```python
from build123d import *
from build123d import SkipClean  # not in build123d's __all__

# Parameters (mm, degrees)
F1_DEPTH = 25
F0_R     = 3
F2_DEPTH = 4
F3_SIZE2 = 24.99999
F3_SIZE  = 19.99999
F4_R     = 1


# Not quite as in the source:
# - a fillet or chamfer is up to 0.001 mm smaller than in the source, because OpenCascade refuses the exact size


with BuildPart() as f1:
    # F0 (on Top) → F1 (new body)
    with BuildSketch(Plane.XY):
        with BuildLine():
            ThreePointArc((2, 16.6805275696), (11.8793939239, 11.8793939239), (16.6805275696, 2))
            Line((16.6805275696, 2), (19.6987309236, 2))
            ThreePointArc((19.6987309236, 2), (14.0007142675, 14.0007142675), (2, 19.6987309236))
            Line((2, 19.6987309236), (2, 16.6805275696))
        make_face()
        with BuildLine():
            ThreePointArc((-2, 16.6805275696), (0, 16.8), (2, 16.6805275696))
            Line((2, 16.6805275696), (2, 19.6987309236))
            ThreePointArc((2, 19.6987309236), (0, 19.8), (-2, 19.6987309236))
            Line((-2, 19.6987309236), (-2, 16.6805275696))
        make_face()
        with BuildLine():
            ThreePointArc((-16.6805275696, 2), (-11.8793939239, 11.8793939239), (-2, 16.6805275696))
            Line((-2, 16.6805275696), (-2, 19.6987309236))
            ThreePointArc((-2, 19.6987309236), (-14.0007142675, 14.0007142675), (-19.6987309236, 2))
            Line((-19.6987309236, 2), (-16.6805275696, 2))
        make_face()
        with BuildLine():
            ThreePointArc((-16.6805275696, -2), (-16.8, 0), (-16.6805275696, 2))
            Line((-16.6805275696, 2), (-19.6987309236, 2))
            ThreePointArc((-19.6987309236, 2), (-19.8, 0), (-19.6987309236, -2))
            Line((-19.6987309236, -2), (-16.6805275696, -2))
        make_face()
        with BuildLine():
            Line((-2, -19.6987309236), (-2, -16.6805275696))
            ThreePointArc((-2, -16.6805275696), (-11.8793939239, -11.8793939239), (-16.6805275696, -2))
            Line((-16.6805275696, -2), (-19.6987309236, -2))
            ThreePointArc((-19.6987309236, -2), (-14.0007142675, -14.0007142675), (-2, -19.6987309236))
        make_face()
        with BuildLine():
            Line((2, -19.6987309236), (2, -16.6805275696))
            ThreePointArc((2, -16.6805275696), (0, -16.8), (-2, -16.6805275696))
            Line((-2, -16.6805275696), (-2, -19.6987309236))
            ThreePointArc((-2, -19.6987309236), (0, -19.8), (2, -19.6987309236))
        make_face()
        with BuildLine():
            Line((19.6987309236, -2), (16.6805275696, -2))
            ThreePointArc((16.6805275696, -2), (11.8793939239, -11.8793939239), (2, -16.6805275696))
            Line((2, -16.6805275696), (2, -19.6987309236))
            ThreePointArc((2, -19.6987309236), (14.0007142675, -14.0007142675), (19.6987309236, -2))
        make_face()
        with BuildLine():
            ThreePointArc((16.6805275696, 2), (16.7701052944, 1.0017826188), (16.8, 0))
            ThreePointArc((16.8, 0), (16.7701052944, -1.0017826188), (16.6805275696, -2))
            Line((16.6805275696, -2), (19.6987309236, -2))
            ThreePointArc((19.6987309236, -2), (19.7746665242, -1.0012811076), (19.8, 0))
            ThreePointArc((19.8, 0), (19.7746665242, 1.0012811076), (19.6987309236, 2))
            Line((19.6987309236, 2), (16.6805275696, 2))
        make_face()
        with BuildLine():
            ThreePointArc((-19.6987309236, -2), (-19.8, 0), (-19.6987309236, 2))
            Line((-19.6987309236, 2), (-39.9499687109, 2))
            ThreePointArc((-39.9499687109, 2), (-39.9874902215, 1.0003128423), (-40, 0))
            ThreePointArc((-40, 0), (-39.9874902215, -1.0003128423), (-39.9499687109, -2))
            Line((-39.9499687109, -2), (-19.6987309236, -2))
        make_face()
        with BuildLine():
            Line((2, -39.9499687109), (2, -19.6987309236))
            ThreePointArc((2, -19.6987309236), (0, -19.8), (-2, -19.6987309236))
            Line((-2, -19.6987309236), (-2, -39.9499687109))
            ThreePointArc((-2, -39.9499687109), (-1.0003128423, -39.9874902215), (0, -40))
            ThreePointArc((0, -40), (1.0003128423, -39.9874902215), (2, -39.9499687109))
        make_face()
        with BuildLine():
            Line((39.9499687109, 2), (19.6987309236, 2))
            ThreePointArc((19.6987309236, 2), (19.7746665242, 1.0012811076), (19.8, 0))
            ThreePointArc((19.8, 0), (19.7746665242, -1.0012811076), (19.6987309236, -2))
            Line((19.6987309236, -2), (39.9499687109, -2))
            ThreePointArc((39.9499687109, -2), (39.9874902215, -1.0003128423), (40, 0))
            ThreePointArc((40, 0), (39.9874902215, 1.0003128423), (39.9499687109, 2))
        make_face()
        with BuildLine():
            ThreePointArc((-2, 19.6987309236), (0, 19.8), (2, 19.6987309236))
            Line((2, 19.6987309236), (2, 39.9499687109))
            ThreePointArc((2, 39.9499687109), (1.0003128423, 39.9874902215), (0, 40))
            ThreePointArc((0, 40), (-1.0003128423, 39.9874902215), (-2, 39.9499687109))
            Line((-2, 39.9499687109), (-2, 19.6987309236))
        make_face()
    extrude(amount=F1_DEPTH)

    # F0 (on Top) → F2 (join)
    with BuildSketch(Plane.XY):
        with BuildLine():
            ThreePointArc((-19.6987309236, 2), (-14.0007142675, 14.0007142675), (-2, 19.6987309236))
            Line((-2, 19.6987309236), (-2, 39.9499687109))
            ThreePointArc((-2, 39.9499687109), (-28.2842712475, 28.2842712475), (-39.9499687109, 2))
            Line((-39.9499687109, 2), (-19.6987309236, 2))
        make_face()
        with Locations((-21, 21)):
            Circle(F0_R, mode=Mode.SUBTRACT)
        with BuildLine():
            ThreePointArc((2, 19.6987309236), (14.0007142675, 14.0007142675), (19.6987309236, 2))
            Line((19.6987309236, 2), (39.9499687109, 2))
            ThreePointArc((39.9499687109, 2), (28.2842712475, 28.2842712475), (2, 39.9499687109))
            Line((2, 39.9499687109), (2, 19.6987309236))
        make_face()
        with Locations((21, 21)):
            Circle(F0_R, mode=Mode.SUBTRACT)
        with BuildLine():
            Line((39.9499687109, 2), (19.6987309236, 2))
            ThreePointArc((19.6987309236, 2), (19.7746665242, 1.0012811076), (19.8, 0))
            ThreePointArc((19.8, 0), (19.7746665242, -1.0012811076), (19.6987309236, -2))
            Line((19.6987309236, -2), (39.9499687109, -2))
            ThreePointArc((39.9499687109, -2), (39.9874902215, -1.0003128423), (40, 0))
            ThreePointArc((40, 0), (39.9874902215, 1.0003128423), (39.9499687109, 2))
        make_face()
        with BuildLine():
            ThreePointArc((-2, 19.6987309236), (0, 19.8), (2, 19.6987309236))
            Line((2, 19.6987309236), (2, 39.9499687109))
            ThreePointArc((2, 39.9499687109), (1.0003128423, 39.9874902215), (0, 40))
            ThreePointArc((0, 40), (-1.0003128423, 39.9874902215), (-2, 39.9499687109))
            Line((-2, 39.9499687109), (-2, 19.6987309236))
        make_face()
        with BuildLine():
            Line((39.9499687109, -2), (19.6987309236, -2))
            ThreePointArc((19.6987309236, -2), (14.0007142675, -14.0007142675), (2, -19.6987309236))
            Line((2, -19.6987309236), (2, -39.9499687109))
            ThreePointArc((2, -39.9499687109), (28.2842712475, -28.2842712475), (39.9499687109, -2))
        make_face()
        with Locations((21, -21)):
            Circle(F0_R, mode=Mode.SUBTRACT)
        with BuildLine():
            Line((19.6987309236, -2), (16.6805275696, -2))
            ThreePointArc((16.6805275696, -2), (11.8793939239, -11.8793939239), (2, -16.6805275696))
            Line((2, -16.6805275696), (2, -19.6987309236))
            ThreePointArc((2, -19.6987309236), (14.0007142675, -14.0007142675), (19.6987309236, -2))
        make_face()
        with BuildLine():
            ThreePointArc((16.6805275696, 2), (16.7701052944, 1.0017826188), (16.8, 0))
            ThreePointArc((16.8, 0), (16.7701052944, -1.0017826188), (16.6805275696, -2))
            Line((16.6805275696, -2), (19.6987309236, -2))
            ThreePointArc((19.6987309236, -2), (19.7746665242, -1.0012811076), (19.8, 0))
            ThreePointArc((19.8, 0), (19.7746665242, 1.0012811076), (19.6987309236, 2))
            Line((19.6987309236, 2), (16.6805275696, 2))
        make_face()
        with BuildLine():
            ThreePointArc((2, 16.6805275696), (11.8793939239, 11.8793939239), (16.6805275696, 2))
            Line((16.6805275696, 2), (19.6987309236, 2))
            ThreePointArc((19.6987309236, 2), (14.0007142675, 14.0007142675), (2, 19.6987309236))
            Line((2, 19.6987309236), (2, 16.6805275696))
        make_face()
        with BuildLine():
            Line((2, -19.6987309236), (2, -16.6805275696))
            ThreePointArc((2, -16.6805275696), (0, -16.8), (-2, -16.6805275696))
            Line((-2, -16.6805275696), (-2, -19.6987309236))
            ThreePointArc((-2, -19.6987309236), (0, -19.8), (2, -19.6987309236))
        make_face()
        with BuildLine():
            Line((2, -39.9499687109), (2, -19.6987309236))
            ThreePointArc((2, -19.6987309236), (0, -19.8), (-2, -19.6987309236))
            Line((-2, -19.6987309236), (-2, -39.9499687109))
            ThreePointArc((-2, -39.9499687109), (-1.0003128423, -39.9874902215), (0, -40))
            ThreePointArc((0, -40), (1.0003128423, -39.9874902215), (2, -39.9499687109))
        make_face()
        with BuildLine():
            Line((-2, -19.6987309236), (-2, -16.6805275696))
            ThreePointArc((-2, -16.6805275696), (-11.8793939239, -11.8793939239), (-16.6805275696, -2))
            Line((-16.6805275696, -2), (-19.6987309236, -2))
            ThreePointArc((-19.6987309236, -2), (-14.0007142675, -14.0007142675), (-2, -19.6987309236))
        make_face()
        with BuildLine():
            Line((-2, -39.9499687109), (-2, -19.6987309236))
            ThreePointArc((-2, -19.6987309236), (-14.0007142675, -14.0007142675), (-19.6987309236, -2))
            Line((-19.6987309236, -2), (-39.9499687109, -2))
            ThreePointArc((-39.9499687109, -2), (-28.2842712475, -28.2842712475), (-2, -39.9499687109))
        make_face()
        with Locations((-21, -21)):
            Circle(F0_R, mode=Mode.SUBTRACT)
        with BuildLine():
            ThreePointArc((-19.6987309236, -2), (-19.8, 0), (-19.6987309236, 2))
            Line((-19.6987309236, 2), (-39.9499687109, 2))
            ThreePointArc((-39.9499687109, 2), (-39.9874902215, 1.0003128423), (-40, 0))
            ThreePointArc((-40, 0), (-39.9874902215, -1.0003128423), (-39.9499687109, -2))
            Line((-39.9499687109, -2), (-19.6987309236, -2))
        make_face()
        with BuildLine():
            ThreePointArc((-16.6805275696, -2), (-16.8, 0), (-16.6805275696, 2))
            Line((-16.6805275696, 2), (-19.6987309236, 2))
            ThreePointArc((-19.6987309236, 2), (-19.8, 0), (-19.6987309236, -2))
            Line((-19.6987309236, -2), (-16.6805275696, -2))
        make_face()
        with BuildLine():
            ThreePointArc((-16.6805275696, 2), (-11.8793939239, 11.8793939239), (-2, 16.6805275696))
            Line((-2, 16.6805275696), (-2, 19.6987309236))
            ThreePointArc((-2, 19.6987309236), (-14.0007142675, 14.0007142675), (-19.6987309236, 2))
            Line((-19.6987309236, 2), (-16.6805275696, 2))
        make_face()
        with BuildLine():
            ThreePointArc((-2, 16.6805275696), (0, 16.8), (2, 16.6805275696))
            Line((2, 16.6805275696), (2, 19.6987309236))
            ThreePointArc((2, 19.6987309236), (0, 19.8), (-2, 19.6987309236))
            Line((-2, 19.6987309236), (-2, 16.6805275696))
        make_face()
    with SkipClean():  # cleaning this boolean's faces spoils the solid; the shape is the same uncleaned
        extrude(amount=-F2_DEPTH)

    # F3 (size 20 and 25 in the source; OpenCascade refuses exactly that, so slightly less here)
    f3_edges = [f1.edges().sort_by_distance(p)[0] for p in [
        (-40, 0, 25),
        (0, -40, 25),
        (40, 0, 25),
        (0, 40, 25),
    ]]
    f3_side = f1.faces().sort_by_distance((-29.82435, 0.868629, 25))[0]
    chamfer(f3_edges, length=F3_SIZE, length2=F3_SIZE2, reference=f3_side)

    # F4
    f4_edges = [f1.edges().sort_by_distance(p)[0] for p in [
        (-16.680528, -2, 25),
    ]]
    fillet(f4_edges, radius=F4_R)


solid = f1.part
```
Input: part model. Units: mm. Frame: model coordinates. A direction names the side the tool comes from. Give positions to 0.01 mm unless a question says otherwise; leave off trailing zeros. Loops run counter-clockwise (first coordinate to the right, second up) from the corner with the lowest first, then second, coordinate; pieces in that order, holes last. Notation, with made-up numbers: (18.5, 3.5) -> (25.5, 3.5) arc R22 ccw to (25.5, 9.5) -> close; hole circle Ø5 at (78, 18). An arc over 180 degrees is marked (long way). Use a Markdown table: item, result.
Q1. Pull-direction query (Y, two-part tool) for faces 5 (the flat face through (21, 17, 0)), 6 (the cylindrical face through (18.6, -22.8, -2)), 7 (the cylindrical face through (-14, 14, 12)), 8 (the cylindrical face through (14, -14, 12)); classes: pulls with the +Y half, pulls with the -Y half, needs draft (parallel to the pull), parting line crosses it, or undercut.
Entries:
| item | result |
|---|---|
| face 5 | needs draft |
| face 6 | undercut |
| face 7 | pulls with the +Y half |
| face 8 | pulls with the -Y half |
Q2. Section query A-A, the plane z = 8. Return the cut outline in (x, y).
Entries:
| item | result |
|---|---|
| outline | (-33.54, -2) -> (-19.7, -2) arc R19.8 ccw to (-2, -19.7) -> (-2, -33.54) arc R33.6 ccw to (2, -33.54) -> (2, -19.7) arc R19.8 ccw to (19.7, -2) -> (33.54, -2) arc R33.6 ccw to (33.54, 2) -> (19.7, 2) arc R19.8 ccw to (2, 19.7) -> (2, 33.54) arc R33.6 ccw to (-2, 33.54) -> (-2, 19.7) arc R19.8 ccw to (-19.7, 2) -> (-33.54, 2) arc R33.6 ccw to start; hole circle Ø33.6 at (0, 0) |
Q3. Section query D-D, the plane z = 16.5. Return the cut outline in (x, y), plus the area to 3 significant figures.
Entries:
| item | result |
|---|---|
| outline | (-26.73, -2) -> (-19.7, -2) arc R19.8 ccw to (-2, -19.7) -> (-2, -26.73) arc R26.8 ccw to (2, -26.73) -> (2, -19.7) arc R19.8 ccw to (19.7, -2) -> (26.73, -2) arc R26.8 ccw to (26.73, 2) -> (19.7, 2) arc R19.8 ccw to (2, 19.7) -> (2, 26.73) arc R26.8 ccw to (-2, 26.73) -> (-2, 19.7) arc R19.8 ccw to (-19.7, 2) -> (-26.73, 2) arc R26.8 ccw to start; hole circle Ø33.6 at (0, 0) |
| area | 457 mm² |
Q4. Ray query, probe 1 along Y at (x, z) = (21, -1.45); probe 2 along Z at (x, y) = (-26, 20); probe 3 along X at (y, z) = (-25, 18.5). Return the intervals inside material, ascending. Write a range as from..to.
Entries:
| item | result |
|---|---|
| probe 1 | y = -34.04..-24, -18..18, 24..34.04 |
| probe 2 | z = -4..0 |
| probe 3 | x = -2..2 |
Q5. Access query for faces 1 (the flat face through (-2, -27, 10)), 2 (the flat face through (2, 27, 10)), 3 (the flat face through (-2, 28, 10)), 4 (the flat face through (21, -16, 0)). Directions: +Z, -Z, +X, -X, +Y, -Y. A direction counts if a zero-diameter tool reaches every point of the face in a straight line with its end or side. Return the directions, or none.
Entries:
| item | result |
|---|---|
| face 1 | +Z, -X, -Y |
| face 2 | +Z, +X, +Y |
| face 3 | +Z, -X, +Y |
| face 4 | +Z, +X, -Y |
Q6. Section query B-B, the plane y = -21. State how many separate pieces and enclosed holes the cut face has, plus the area to 3 significant figures.
Entries:
| item | result |
|---|---|
| separate pieces | 3 |
| enclosed holes | 0 |
| area | 319 mm² |
Q7. First-contact query: P1, Ø1, axis at y = -13.5, z = 14, coming from the +X side; P2, Ø10, axis at y = 25, z = 11, coming from the +X side; P3, Ø8, axis at x = 24.5, z = 21.5, coming from the -Y side; P4, Ø9.5, axis at x = -21, y = 21, coming from the -Z side. Flat tips, straight axial feed; report the tip coordinate or a pass-through.
Entries:
| item | result |
|---|---|
| P1 | stops at x = 14.93 |
| P2 | stops at x = 2 |
| P3 | stops at y = -2 |
| P4 | stops at z = -4 |
